Drawing for the job (mm, zero at the part's lowest x, y, z). A direction names the side the tool comes from. Round coordinates to 2 decimals unless told otherwise and drop trailing zeros. Loops run counter-clockwise (first coordinate to the right, second up) from the corner with the lowest first, then second, coordinate; pieces in that order, holes last. Notation, with made-up numbers: (84, 48.25) -> (93, 48.25) arc R16 ccw to (93, 64.25) -> close; hole circle Ø4 at (7, 52). An arc over 180 degrees is marked (long way). Put each result on its own line as item: value. Start each with the question number.
Item 1: Flat gauge pins, fed straight in: pin 1 Ø1.2 at (x, z) = (36.5, 6.5) entering from -Y; pin 2 Ø6.5 at (x, z) = (37, 4) entering from +Y; pin 3 Ø2 at (y, z) = (9.5, 10.5) entering from +X. Where does each tip first touch, or does it go through?
Item 2: Cut at C-C, the plane x = 3.25. List the corners of the cut face in (y, z).
Item 3: Cut at B-B, the plane y = 19.5. List the corners of the cut face in (x, z), plus the area to 3 significant figures.
Item 4: Cut at A-A, the plane x = 28.5. List the corners of the cut face in (y, z).
Item 5: Drill centre lines: probe 1 along Y at (x, z) = (14, 6); probe 2 along Y at (x, z) = (10, 6.25); probe 3 along X at (y, z) = (31.5, 9). Where is each one in solid material? Low to high. Write a range as [from, to].
Item 6: Cut at D-D, the plane z = 7.5. List the corners of the cut face in (x, y), plus the area to 3 significant figures.
Item 7: Tool access for the marked faces 1, 2, 3 and 4: list every direction of +Z, -Z, +X, -X, +Y, -Y with a clear straight run to the whole face (end or side of a thin tool).
Item 8: Pull direction X, two halves, no side cores. Call the marked faces 5, 6, 7 and 8: +X half, -X half, draft (parallel to the pull), parting line (faces both ways), or undercut.
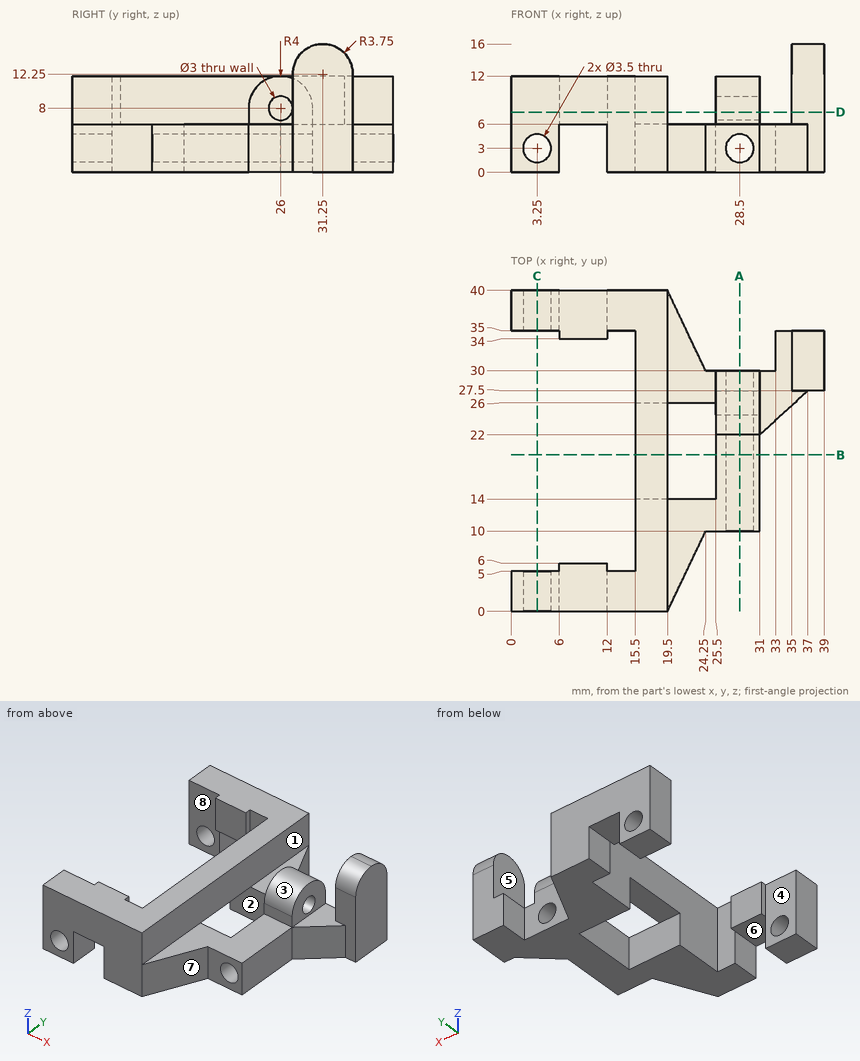
Reply:
1. pin 1: stops at y = 26.74
1. pin 2: stops at y = 35
1. pin 3: stops at x = 19.5
2. outline: (0, 0) -> (5, 0) -> (5, 1.25) -> (0, 1.25) -> close; (0, 4.75) -> (5, 4.75) -> (5, 12) -> (0, 12) -> close; (35, 0) -> (40, 0) -> (40, 1.25) -> (35, 1.25) -> close; (35, 4.75) -> (40, 4.75) -> (40, 12) -> (35, 12) -> close
3. outline: (15.5, 6) -> (19.5, 6) -> (19.5, 12) -> (15.5, 12) -> close; (25.5, 0) -> (31, 0) -> (31, 6) -> (25.5, 6) -> close; hole circle Ø3.5 at (28.5, 3)
3. area: 47.4 mm^2
4. outline: (10, 0) -> (30, 0) -> (30, 1.25) -> (10, 1.25) -> close; (10, 4.75) -> (30, 4.75) -> (30, 8) arc R4 ccw to (22, 8) -> (22, 6) -> (10, 6) -> close; hole circle Ø3 at (26, 8)
5. probe 1: y = [0, 5], [35, 40]
5. probe 2: y = [0, 6], [34, 40]
5. probe 3: x = [15.5, 19.5], [35, 39]
6. outline: (0, 0) -> (19.5, 0) -> (19.5, 40) -> (0, 40) -> (0, 35) -> (6, 35) -> (6, 34) -> (12, 34) -> (12, 35) -> (15.5, 35) -> (15.5, 5) -> (12, 5) -> (12, 6) -> (6, 6) -> (6, 5) -> (0, 5) -> close; (25.5, 22) -> (31, 22) -> (31, 24.59) -> (25.5, 24.59) -> close; (25.5, 27.41) -> (31, 27.41) -> (31, 30) -> (25.5, 30) -> close; (35, 27.5) -> (39, 27.5) -> (39, 35) -> (35, 35) -> close
6. area: 385 mm^2
7. face 1: +Z, +Y, -Y
7. face 2: -Z, -X
7. face 3: +Z
7. face 4: +Z, -Z, -X
8. face 5: undercut
8. face 6: undercut
8. face 7: +X half
8. face 8: draft
